Read the model definition and answer for the solid it produces. Units are mm, in the model's axes. A direction names the side the tool comes from. Round coordinates to 2 decimals unless told otherwise and drop trailing zeros. Order: outer loops, then holes, each group sorted by start corner. A loop starts at its lowest first (then second) coordinate and runs counter-clockwise, first axis right, second up.
Autodesk Inventor part; units mm, degrees
ref_plane "YZ Plane" through (0, 0, 0) normal (1, 0, 0) x (0, 1, 0)
ref_plane "XZ Plane" through (0, 0, 0) normal (0, 1, 0) x (-1, 0, 0)
ref_plane "XY Plane" through (0, 0, 0) normal (0, 0, 1) x (1, 0, 0)
sketch "Sketch2" plane through (0, 0, 0) normal (0, 1, 0) x (-1, 0, 0)
  circle A0 centre (0, 0) radius 34.925
  line L0 (0, 0) -> (0, -38.1)
  line L1 (0, -38.1) -> (-14.1986, -38.1)
  line L2 (-14.1986, -38.1) -> (14.1986, -38.1)
  circle A1 centre (14.1986, -38.1) radius 2.159
  circle A2 centre (-14.1986, -38.1) radius 2.159
  circle A3 centre (-14.1986, -38.1) radius 4.2333
  line L3 (-14.1986, -38.1) -> (-14.1986, 44.45) construction
  line L4 (-9.9653, -38.1) -> (-9.9653, 44.45)
  line L5 (-18.4319, 44.45) -> (-18.4319, -38.1)
  arc A4 (-18.4319, -38.1) -> (-9.9653, -38.1) centre (-14.1986, -38.1) ccw
  arc A5 (-9.9653, 44.45) -> (-18.4319, 44.45) centre (-14.1986, 44.45) ccw
  line L6 (-14.1986, 44.45) -> (33.4617, -38.1) construction
  line L7 (-17.8648, 42.3333) -> (29.7955, -40.2167)
  line L8 (37.1278, -35.9833) -> (-10.5324, 46.5667)
  arc A6 (-10.5324, 46.5667) -> (-17.8648, 42.3333) centre (-14.1986, 44.45) ccw
  arc A7 (29.7955, -40.2167) -> (37.1278, -35.9833) centre (33.4617, -38.1) ccw
  line L9 (-14.1986, 44.45) -> (81.1219, 44.45) construction
  line L10 (-14.1986, -38.1) -> (33.4617, -38.1) construction
  line L11 (-14.1986, -33.8667) -> (33.4617, -33.8667)
  line L12 (33.4617, -42.3333) -> (-14.1986, -42.3333)
  arc A8 (-14.1986, -33.8667) -> (-14.1986, -42.3333) centre (-14.1986, -38.1) ccw
  arc A9 (33.4617, -42.3333) -> (33.4617, -33.8667) centre (33.4617, -38.1) ccw
  point P0 (-14.1986, 3.175)
  point P1 (9.6315, 3.175)
  point P2 (9.6315, -38.1)
  point P3 (-9.9653, 28.651)
  point P4 (26.1293, -33.8667)
  point P5 (-9.9653, -33.8667)
  point P6 (-18.4319, -38.1)
  dimension "d17" = 69.85
  dimension "d18" = 38.1
  dimension "d19" = 14.1986
  dimension "d20" = 28.3972
  dimension "d21" = 4.318
  dimension "d22" = 4.318
  dimension "d23" = 8.4667
  dimension "d24" = 82.55
  dimension "d25" = 8.4667
  dimension "d26" = 60
  dimension "d27" = 8.4667
extrude "Extrusion2" add sketch "Sketch2" along normal blind 1.5875 contours L8 A0 L7 L4 | A0 L4 A5 L8 | L8 A9 L11 L7 A0 | L4 L7 A0 | A0 L7 A6 A5 L4 | A7 L7 L11 A9 | L7 L4 A0 L5 | A0 L5 A6 L7 | L11 L7 A7 L12 A3 L1 L0 A0 | A0 L0 L11 | L4 L11 A3 L5 A0 | L0 L1 L4 L11 A0 | A0 L11 L0 | A3 | L4 A3 L11
fillet "Fillet4" radius 4.2333 3 edges at (-26.1293, 0.7937, -33.8667) (9.9653, 0.7937, -33.8667) (9.9653, 0.7937, 28.651)
sketch "Sketch3" plane through (0, 1.5875, 0) normal (0, 1, 0) x (1, 0, 0)
  arc A0 (10.5324, -46.5667) -> (18.4319, -44.45) centre (14.1986, -44.45) ccw
  circle A1 centre (14.1986, -44.45) radius 2.159
  point P0 (0, 0)
  dimension "d31" = 4.318
extrude "Extrusion3" cut sketch "Sketch3" against normal blind 1.5875
properties part number "sheet1" material "Acetal Resin, Black"
Q1. A cutting plane is placed at A-A, the plane z = -18. Give the vertices of the cut face in (x, y), plus the area to 3 significant figures.
Outcome:
outline: (-26.75, 0) - (-16.97, 0) - (-16.97, 1.59) - (-26.75, 1.59) - close; (9.97, 0) - (18.43, 0) - (18.43, 1.59) - (9.97, 1.59) - close
area: 29.0 mm2
Q2. A cutting plane is placed at B-B, the plane y = 1.3. Give the vertices of the cut face in (x, z), plus the area to 3 significant figures.
Outcome:
outline: (-37.13, -35.98) arc R4.23 ccw to (-33.46, -42.33) - (14.2, -42.33) arc R4.23 ccw to (18.43, -38.1) - (18.43, 44.45) arc R4.23 ccw to (10.53, 46.57) - close; hole (-22.46, -27.52) arc R4.23 ccw to (-18.8, -33.87) - (5.73, -33.87) arc R4.23 ccw to (9.97, -29.63) - (9.97, 12.85) arc R4.23 ccw to (2.07, 14.97) - close; hole circle Ø4.32 at (-14.2, -38.1); hole circle Ø4.32 at (14.2, -38.1); hole circle Ø4.32 at (14.2, 44.45)
area: 1,870 mm2
Q3. A cutting plane is placed at C-C, the plane z = 23. Give the vertices of the cut face in (x, y).
Outcome:
outline: (-3.07, 0) - (18.43, 0) - (18.43, 1.59) - (-3.07, 1.59) - close
Q4. For a pull along X with two mould halves and no side action, classify faces 1 (the face through (14.7, 0.8, -36)), 2 (the face through (-13.631, 0.783, 4.714)), 3 (the face through (15.37, 0.78, 48.52)) as released by +X, released by -X, zero draft, split by the parting line, or undercut.
Outcome:
face 1: undercut
face 2: released by -X
face 3: split by the parting line
Q5. For faces 4 (the face through (-37.16, 0.78, -40.16)), 5 (the face through (6.75, 0.8, 16.96)), determine the directions among +Z, -Z, +X, -X, +Y, -Y from which every point of the face is accessible in a straight line to the end or side of a thin tool.
Outcome:
face 4: -X, +Y, -Y
face 5: +Y, -Y
Q6. A flat-ended cylindrical pin translates along its axis: pin 1 (5 mm diameter, centred on x = -14.2, z = -38.1, fed in from -Y). Find the tip coordinate at first contact, or state that the pin passes through.
Outcome:
pin 1: stops at y = 0
Q7. A cutting plane is placed at D-D, the plane x = -30. Give the vertices of the cut face in (y, z).
Outcome:
outline: (0, -42.33) - (1.59, -42.33) - (1.59, -23.64) - (0, -23.64) - close
Q8. Straight lines are drawn through the part: probe 1 along Z at (x, y) = (-14, 0.95); probe 2 along X at (y, z) = (1.35, -38); probe 3 along Z at (x, y) = (14.5, 0.8). For each, find the intervals that lie inside material, in ascending order.
Outcome:
probe 1: z = -42.33 to -40.25, -35.95 to -33.87, -12.86 to 4.08
probe 2: x = -37.69 to -16.36, -12.04 to 12.04, 16.36 to 18.43
probe 3: z = -42.32 to -40.24, -35.96 to 42.31, 46.59 to 48.67
